Can you work these out from the drawing? Everything is in mm from the part's minimum corner. A direction names the side the tool comes from. Round coordinates to 2 decimals unless told otherwise and drop trailing zeros. Order: outer loops, then holes, each group sorted by start corner. A loop starts at its lowest first (then second) coordinate and runs counter-clockwise, first axis right, second up. Notation, with made-up numbers: M -3.75,30.25 L 23.25,30.25 A17 ccw 23.25,60.25 Z; hole C 36,29.25 d4. An arc over 180 degrees is marked long. Write item = value, one per line. Start each with the question number.
Item 1: I'm going to push flat-ended pins straight in: P1, Ø4.5, axis at x = 23.5, z = 19, coming from the +Y side; P2, Ø8.5, axis at x = 40, z = 20, coming from the -Y side. Where does each tip first touch, or does it pass through?
Item 2: I want a section at C-C, the plane z = 20. List the corners of the cut face in (x, y) for me.
Item 3: I want a section at A-A, the plane x = 40. List the corners of the cut face in (y, z) for me, plus the area to 3 significant figures.
Item 4: I want a section at D-D, the plane x = 60. List the corners of the cut face in (y, z) for me, plus the area to 3 significant figures.
Item 5: Please list where these lines run through material, in increasing order: L1, parallel to X at y = 5.25, z = 20; L2, parallel to Z at x = 40, y = 10.25; L3, parallel to Z at x = 60, y = 7.75.
Item 6: For the marked faces 4 and 5, which set-ups out of +Z, -Z, +X, -X, +Y, -Y let a thin tool reach every point of the face, with its end or its side?
Item 7: I want a section at B-B, the plane y = 3.75. List the corners of the cut face in (x, z) for me.
Item 8: We'd pull the mould along X, two halves only. Please class the marked faces 1, 2 and 3: pulls with the +X half, pulls with the -X half, needs draft (parallel to the pull), parting line crosses it, or undercut.
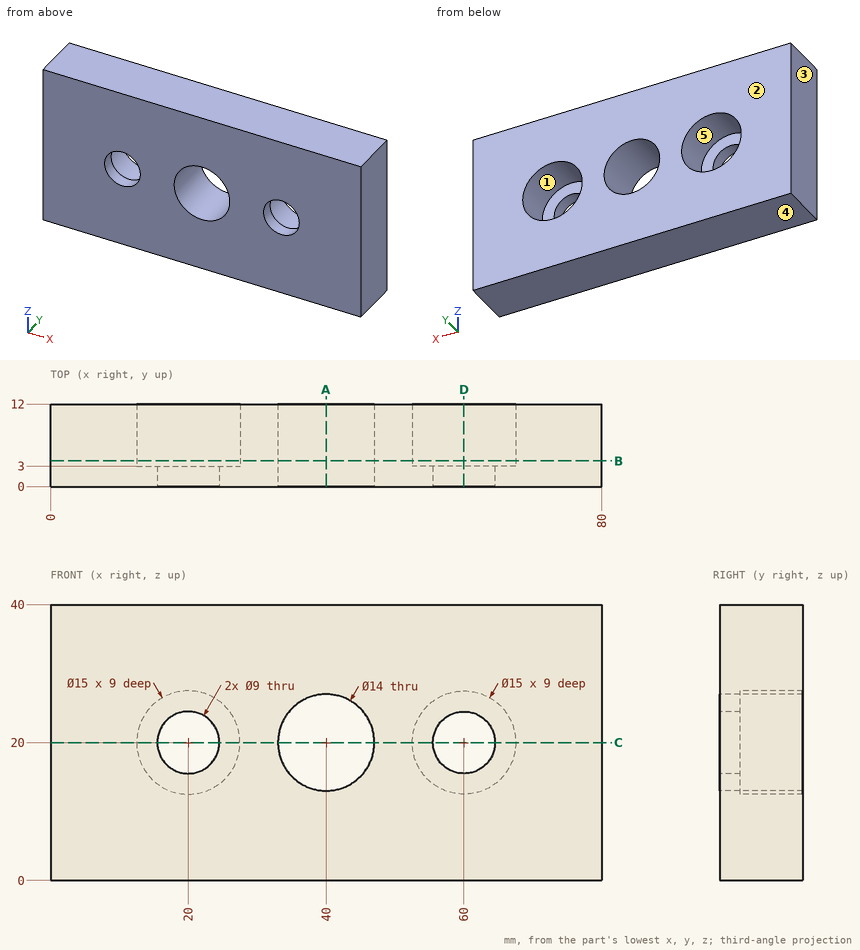
Filled in:
q1.P1 = 3
q1.P2 = through
q2.outline = M 0,0 L 15.5,0 L 15.5,3 L 12.5,3 L 12.5,12 L 0,12 Z; M 24.5,0 L 33,0 L 33,12 L 27.5,12 L 27.5,3 L 24.5,3 Z; M 47,0 L 55.5,0 L 55.5,3 L 52.5,3 L 52.5,12 L 47,12 Z; M 64.5,0 L 80,0 L 80,12 L 67.5,12 L 67.5,3 L 64.5,3 Z
q3.outline = M 0,0 L 12,0 L 12,13 L 0,13 Z; M 0,27 L 12,27 L 12,40 L 0,40 Z
q3.area = 312 mm^2
q4.outline = M 0,0 L 12,0 L 12,12.5 L 3,12.5 L 3,15.5 L 0,15.5 Z; M 0,24.5 L 3,24.5 L 3,27.5 L 12,27.5 L 12,40 L 0,40 Z
q4.area = 318 mm^2
q5.L1 = 0 to 12.5, 27.5 to 33, 47 to 52.5, 67.5 to 80
q5.L2 = 0 to 13, 27 to 40
q5.L3 = 0 to 12.5, 27.5 to 40
q6.face_4 = -Z, +X, -X, +Y, -Y
q6.face_5 = +Y
q7.outline = M 0,0 L 80,0 L 80,40 L 0,40 Z; hole C 20,20 d15; hole C 40,20 d14; hole C 60,20 d15
q8.face_1 = undercut
q8.face_2 = needs draft
q8.face_3 = pulls with the -X half
